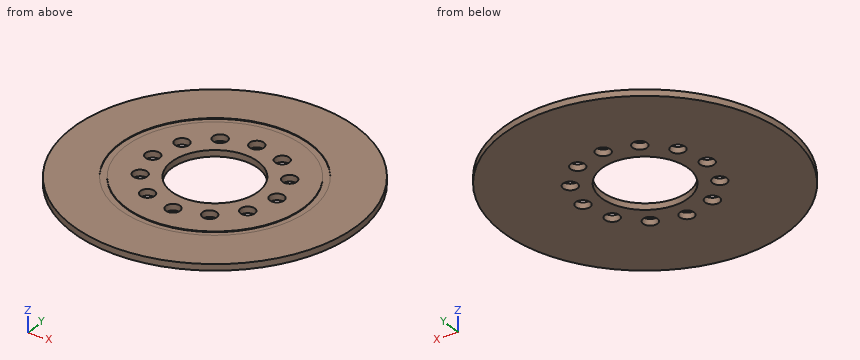
```python
from build123d import *

# Parameters (mm, degrees)
SKETCH1_R           = 79
BOSS_EXTRUDE1_DEPTH = 3.5
SKETCH2_R           = 4
SKETCH2_R_2         = 24.1
CUT_EXTRUDE1_DEPTH  = 112.777681135
SKETCH3_R           = 53
SKETCH3_R_2         = 49.5
CUT_EXTRUDE2_DEPTH  = 0.4


with BuildPart() as part:
    # Sketch1 → Boss-Extrude1 (new body)
    with BuildSketch(Plane.XY):
        Circle(SKETCH1_R)
    extrude(amount=BOSS_EXTRUDE1_DEPTH)

    # Sketch2 → Cut-Extrude1 (cut, through all)
    with BuildSketch(Plane.XY):
        with Locations((34.4, 0)):
            Circle(SKETCH2_R)
        with Locations((29.79127389, -17.2)):
            Circle(SKETCH2_R)
        with Locations((17.2, -29.79127389)):
            Circle(SKETCH2_R)
        with Locations((0, -34.4)):
            Circle(SKETCH2_R)
        with Locations((-17.2, -29.79127389)):
            Circle(SKETCH2_R)
        with Locations((-29.79127389, -17.2)):
            Circle(SKETCH2_R)
        with Locations((-34.4, 0)):
            Circle(SKETCH2_R)
        with Locations((-29.79127389, 17.2)):
            Circle(SKETCH2_R)
        with Locations((-17.2, 29.79127389)):
            Circle(SKETCH2_R)
        with Locations((0, 34.4)):
            Circle(SKETCH2_R)
        with Locations((17.2, 29.79127389)):
            Circle(SKETCH2_R)
        with Locations((29.79127389, 17.2)):
            Circle(SKETCH2_R)
        Circle(SKETCH2_R_2)
    extrude(amount=CUT_EXTRUDE1_DEPTH, mode=Mode.SUBTRACT)

    # Sketch3 → Cut-Extrude2 (cut)
    with BuildSketch(Plane.XY.offset(3.5)):
        Circle(SKETCH3_R)
        Circle(SKETCH3_R_2, mode=Mode.SUBTRACT)
    extrude(amount=-CUT_EXTRUDE2_DEPTH, mode=Mode.SUBTRACT)


solid = part.part
```
Here's how the part is built. I have some questions about the finished solid (model axes, mm). Coordinates: 2 decimals unless noted, no trailing zeros. Order: outer loops, then holes, each group sorted by start corner. A loop starts at its lowest first (then second) coordinate and runs counter-clockwise, first axis right, second up. Notation, with made-up numbers: (-19, 55) - (32, 55) arc R10 ccw to (32, 60) - close; hole circle Ø5 at (4.5, 45). An arc over 180 degrees is marked (long way). One line per question, with ' | ' between items.
(1) Suppose I cut it at D-D on y = -62. List the corners of the cut face in (x, z) for me.
Report:
outline: (-48.96, 0) - (48.96, 0) - (48.96, 3.5) - (-48.96, 3.5) - close
(2) Suppose I cut it at B-B on x = -17.2. List the corners of the cut face in (y, z) for me, and give its area (3 significant figures).
Report:
outline: (-77.1, 0) - (-33.79, 0) - (-33.79, 3.5) - (-46.42, 3.5) - (-46.42, 3.1) - (-50.13, 3.1) - (-50.13, 3.5) - (-77.1, 3.5) - close; (-25.79, 0) - (-16.88, 0) - (-16.88, 3.5) - (-25.79, 3.5) - close; (16.88, 0) - (25.79, 0) - (25.79, 3.5) - (16.88, 3.5) - close; (33.79, 0) - (77.1, 0) - (77.1, 3.5) - (50.13, 3.5) - (50.13, 3.1) - (46.42, 3.1) - (46.42, 3.5) - (33.79, 3.5) - close | area: 363 mm2
(3) Will these pins go through, and if not, where does the flat tip stop? pin 1 (5 mm diameter, centred on x = -34.4, y = 0, fed in from +Z); pin 2 (13 mm diameter, centred on x = 0, y = 34.4, fed in from +Z); pin 3 (2 mm diameter, centred on x = 24.5, z = 1, fed in from +Y).
Report:
pin 1: passes through | pin 2: stops at z = 3.5 | pin 3: stops at y = 75.42
(4) Suppose I cut it at C-C on z = 1.7. State how many separate pieces and enclosed holes the cut face has, and give its area (3 significant figures).
Report:
separate pieces: 1 | enclosed holes: 13 | area: 17,200 mm2
(5) If I drill on L1, parallel to Y at x = 0, z = 3.35; L2, parallel to Y at x = 0, z = 1.2; L3, parallel to X at y = 17.2, z = 1.75, over which ranges is the centre line in solid material (lowest first)?
Report:
L1: y = -79 to -53, -49.5 to -38.4, -30.4 to -24.1, 24.1 to 30.4, 38.4 to 49.5, 53 to 79 | L2: y = -79 to -38.4, -30.4 to -24.1, 24.1 to 30.4, 38.4 to 79 | L3: x = -77.1 to -33.79, -25.79 to -16.88, 16.88 to 25.79, 33.79 to 77.1
(6) Suppose I cut it at A-A on y = 0. List the corners of the cut face in (x, z) for me, and give its area (4 significant figures).
Report:
outline: (-79, 0) - (-38.4, 0) - (-38.4, 3.5) - (-49.5, 3.5) - (-49.5, 3.1) - (-53, 3.1) - (-53, 3.5) - (-79, 3.5) - close; (-30.4, 0) - (-24.1, 0) - (-24.1, 3.5) - (-30.4, 3.5) - close; (24.1, 0) - (30.4, 0) - (30.4, 3.5) - (24.1, 3.5) - close; (38.4, 0) - (79, 0) - (79, 3.5) - (53, 3.5) - (53, 3.1) - (49.5, 3.1) - (49.5, 3.5) - (38.4, 3.5) - close | area: 325.5 mm2
